Can you work these out from the model? Positions are in its coordinate system, mm. Face numbers are marked on the shaded views. A direction names the side the tool comes from. Round coordinates to 2 decimals unless told otherwise and drop trailing zeros. Loops run counter-clockwise (first coordinate to the right, second up) from the corner with the lowest first, then second, coordinate; pieces in that order, holes last. Notation, with made-up numbers: M 88,68 L 96,68 A15 ccw 96,91 Z; hole C -16,73 d3. An arc over 180 degrees is marked long. Answer as CSV lines item,"result".
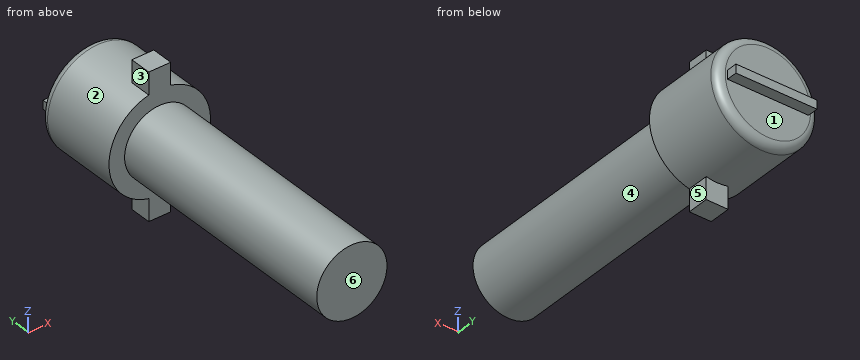
from build123d import *

# Parameters (mm, degrees)
SKETCH1_R           = 3.25
BOSS_EXTRUDE1_DEPTH = 22.686
SKETCH6_R           = 4.7
BOSS_EXTRUDE2_DEPTH = 8
BOSS_EXTRUDE3_DEPTH = 1
FILLET1_R           = 0.75
SKETCH9_W           = 0.8
SKETCH9_H           = 3.35
CUT_EXTRUDE3_DEPTH  = 1
BOSS_EXTRUDE4_DEPTH = 2


with BuildPart() as part:
    # Sketch1 → Boss-Extrude1 (new body)
    with BuildSketch(Plane(origin=(0, 0, 0), x_dir=(1, 0, 0), z_dir=(0, 1, 0))):
        Circle(SKETCH1_R)
    extrude(amount=BOSS_EXTRUDE1_DEPTH)

    # Sketch6 → Boss-Extrude2 (add)
    with BuildSketch(Plane(origin=(0, 22.686, 0), x_dir=(1, 0, 0), z_dir=(0, 1, 0))):
        Circle(SKETCH6_R)
    extrude(amount=BOSS_EXTRUDE2_DEPTH)

    # Sketch8 → Boss-Extrude3 (add)
    with BuildSketch(Plane(origin=(0, 30.686, 0), x_dir=(1, 0, 0), z_dir=(0, 1, 0))):
        Polygon((0.4, 3.75), (-0.4, 3.75), (-0.4, 0.4), (-3.75, 0.4), (-3.75, -0.4), (-0.4, -0.4), (-0.4, -3.75), (0.4, -3.75), (0.4, -0.4), (3.75, -0.4), (3.75, 0.4), (0.4, 0.4), align=None)
    extrude(amount=BOSS_EXTRUDE3_DEPTH)

    # Fillet1
    fillet1_edges = [part.edges().sort_by_distance(p)[0] for p in [
        (-4.7, 30.686, 0),
    ]]
    fillet(fillet1_edges, radius=FILLET1_R)

    # Sketch9 → Cut-Extrude3 (cut)
    with BuildSketch(Plane(origin=(0, 30.686, 0), x_dir=(1, 0, 0), z_dir=(0, 1, 0))):
        with Locations((0, 2.075)):
            Rectangle(SKETCH9_W, SKETCH9_H)
        with Locations((0, -2.075)):
            Rectangle(SKETCH9_W, SKETCH9_H)
    extrude(amount=CUT_EXTRUDE3_DEPTH, mode=Mode.SUBTRACT)

    # Sketch10 → Boss-Extrude4 (add)
    with BuildSketch(Plane.XZ.offset(-22.686)):
        with BuildLine():
            Line((-1.016, 6.620871757), (-1.016, 4.588871757))
            ThreePointArc((-1.016, 4.588871757), (0, 4.7), (1.016, 4.588871757))
            Line((1.016, 4.588871757), (1.016, 6.620871757))
            Line((1.016, 6.620871757), (-1.016, 6.620871757))
        make_face()
        with BuildLine():
            ThreePointArc((1.016, -4.588871757), (0, -4.7), (-1.016, -4.588871757))
            Line((-1.016, -4.588871757), (-1.016, -6.620871757))
            Line((-1.016, -6.620871757), (1.016, -6.620871757))
            Line((1.016, -6.620871757), (1.016, -4.588871757))
        make_face()
    extrude(amount=-BOSS_EXTRUDE4_DEPTH)


solid = part.part
Item 1: Will these pins go through, and if not, where does the flat tip stop? pin 1 (0.6 mm diameter, centred on y = 23.5, z = 6, fed in from +X); pin 2 (2 mm diameter, centred on x = 0, z = -6, fed in from +Y); pin 3 (0.6 mm diameter, centred on y = 23.5, z = -5, fed in from -X).
Output:
pin 1,"stops at x = 1.02"
pin 2,"stops at y = 24.69"
pin 3,"stops at x = -1.02"
Item 2: If we section it at D-D on z = 5.25: Write out the boundary of the cut face in (x, y).
Output:
outline,"M -1.02,22.69 L 1.02,22.69 L 1.02,24.69 L -1.02,24.69 Z"
Item 3: If we section it at A-A on z = 0: Write out the boundary of the cut face in (x, y).
Output:
outline,"M -4.7,22.69 L -3.25,22.69 L -3.25,0 L 3.25,0 L 3.25,22.69 L 4.7,22.69 L 4.7,29.94 A0.75 ccw 3.95,30.69 L 3.75,30.69 L 3.75,31.69 L -3.75,31.69 L -3.75,30.69 L -3.95,30.69 A0.75 ccw -4.7,29.94 Z"
Item 4: If we section it at B-B on x = 0: Write out the boundary of the cut face in (y, z), then the cut area to 3 significant figures.
Output:
outline,"M 0,-3.25 L 22.69,-3.25 L 22.69,-6.62 L 24.69,-6.62 L 24.69,-4.7 L 29.94,-4.7 A0.75 ccw 30.69,-3.95 L 30.69,-0.4 L 31.69,-0.4 L 31.69,0.4 L 30.69,0.4 L 30.69,3.95 A0.75 ccw 29.94,4.7 L 24.69,4.7 L 24.69,6.62 L 22.69,6.62 L 22.69,3.25 L 0,3.25 Z"
area,"231 mm2"
Item 5: If I drill on line 1 along Z through (x, y) = (-0.25, 28); line 2 along Y through (x, z) = (0.5, 2.75); line 3 along Y through (x, z) = (-0.5, 5.5), over which ranges is the centre line in solid material (lowest first)? Write a range as from..to.
Output:
line 1,"z = -4.69..4.69"
line 2,"y = 0..30.69"
line 3,"y = 22.69..24.69"
Item 6: We'd pull the mould along X, two halves only. Please class the marked faces 1, 2 and 3: released by +X, released by -X, zero draft, split by the parting line, or undercut.
Output:
face 1,"zero draft"
face 2,"split by the parting line"
face 3,"released by -X"
Item 7: If we section it at C-C on y = 23.5: Write out the boundary of the cut face in (x, z).
Output:
outline,"M -1.02,-6.62 L 1.02,-6.62 L 1.02,-4.59 A4.7 ccw 1.02,4.59 L 1.02,6.62 L -1.02,6.62 L -1.02,4.59 A4.7 ccw -1.02,-4.59 Z"
Item 8: On a 3-axis mill with a long thin cutter (end or side, diameter ignored), from which of +Z, -Z, +X, -X, +Y, -Y can I reach the whole of each face in a straight line? I mean the marked faces 4, 5 and 6. Say none if no direction works.
Output:
face 4,"-Y"
face 5,"-Z, +X, +Y, -Y"
face 6,"+Z, -Z, +X, -X, -Y"
